from build123d import *

# Parameters (mm, degrees)
PAD_DEPTH       = 10
PAD003_DEPTH    = 12
POCKET_DEPTH    = 10
PAD004_DEPTH    = 12
POCKET004_DEPTH = 2
POCKET001_DEPTH = 10.001
SKETCH004_W     = 160
SKETCH004_H     = 60
PAD002_DEPTH    = 10
SKETCH005_W     = 156
SKETCH005_H     = 56
PAD005_DEPTH    = 12
SKETCH009_W     = 152
SKETCH009_H     = 52
POCKET006_DEPTH = 10
SKETCH006_W     = 18
SKETCH006_H     = 12
POCKET005_DEPTH = 10


with BuildPart() as part:
    # Sketch001 → Pad (new body)
    with BuildSketch(Plane.XY):
        with BuildLine():
            ThreePointArc((0, 57.236352), (-106.486482, 50.845622), (-101.68, -55.72412))
            Line((-101.68, -55.72412), (0, -150.0248))
            Line((0, -150.0248), (101.68, -55.72412))
            ThreePointArc((101.68, -55.72412), (106.486482, 50.845622), (0, 57.236352))
        make_face()
    extrude(amount=PAD_DEPTH)

    # Sketch002 → Pad003 (join)
    with BuildSketch(Plane.XY):
        with BuildLine():
            ThreePointArc((0, 54.552727), (-104.405447, 50.160217), (-100.32, -54.257696))
            Line((-100.32, -54.257696), (0, -147.297076))
            Line((0, -147.297076), (100.32, -54.257696))
            ThreePointArc((100.32, -54.257696), (104.405447, 50.160217), (0, 54.552727))
        make_face()
    extrude(amount=PAD003_DEPTH)

    # Sketch007 → Pocket (cut)
    with BuildSketch(Plane.XY.offset(12)):
        with BuildLine():
            ThreePointArc((0, 51.807335), (-102.301889, 49.482446), (-98.96, -52.791272))
            Line((-98.96, -52.791272), (0, -144.569352))
            Line((0, -144.569352), (98.96, -52.791272))
            ThreePointArc((98.96, -52.791272), (102.301889, 49.482446), (0, 51.807335))
        make_face()
    extrude(amount=-POCKET_DEPTH, mode=Mode.SUBTRACT)

    # Sketch008 → Pad004 (join)
    with BuildSketch(Plane.XY):
        with BuildLine():
            ThreePointArc((0, 33.166248), (-88.852758, 45.721583), (-90.8, -43.992727))
            Line((-90.8, -43.992727), (0, -128.203011))
            Line((0, -128.203011), (90.8, -43.992727))
            ThreePointArc((90.8, -43.992727), (88.852758, 45.721583), (0, 33.166248))
        make_face()
    extrude(amount=PAD004_DEPTH)

    # Sketch003 → Pocket004 (cut)
    with BuildSketch(Plane.XY.offset(12)):
        with BuildLine():
            ThreePointArc((0, 29.393877), (-86.345652, 45.199486), (-89.44, -42.526302))
            Line((-89.44, -42.526302), (0, -125.475287))
            Line((0, -125.475287), (89.44, -42.526302))
            ThreePointArc((89.44, -42.526302), (86.345652, 45.199486), (0, 29.393877))
        make_face()
    extrude(amount=-POCKET004_DEPTH, mode=Mode.SUBTRACT)

    # Sketch → Pocket001 (cut, through all)
    with BuildSketch(Plane.XY.offset(10)):
        with BuildLine():
            ThreePointArc((0, 25.21904), (-83.671135, 44.74656), (-88.08, -41.059878))
            Line((-88.08, -41.059878), (0, -122.747563))
            Line((0, -122.747563), (88.08, -41.059878))
            ThreePointArc((88.08, -41.059878), (83.671135, 44.74656), (0, 25.21904))
        make_face()
    extrude(amount=-POCKET001_DEPTH, mode=Mode.SUBTRACT)

    # Sketch004 → Pad002 (join)
    with BuildSketch(Plane.XY):
        with Locations((0, -170)):
            Rectangle(SKETCH004_W, SKETCH004_H)
    extrude(amount=PAD002_DEPTH)

    # Sketch005 → Pad005 (join)
    with BuildSketch(Plane.XY):
        with Locations((0, -170)):
            Rectangle(SKETCH005_W, SKETCH005_H)
    extrude(amount=PAD005_DEPTH)

    # Sketch009 → Pocket006 (cut)
    with BuildSketch(Plane.XY.offset(12)):
        with Locations((0, -170)):
            Rectangle(SKETCH009_W, SKETCH009_H)
    extrude(amount=-POCKET006_DEPTH, mode=Mode.SUBTRACT)

    # Sketch006 → Pocket005 (cut)
    with BuildSketch(Plane.XY.offset(12)):
        with Locations((0, -142.076699)):
            Rectangle(SKETCH006_W, SKETCH006_H)
    extrude(amount=-POCKET005_DEPTH, mode=Mode.SUBTRACT)


solid = part.part
For this review, take the finished solid that the model builds, in its own axes (mm). A direction names the side the tool comes from. Round coordinates to 2 decimals unless told otherwise and drop trailing zeros. Write each loop counter-clockwise with the first axis right and the second up, starting at its lowest first coordinate (ties: lowest second). Pieces come first, ordered by that corner, then holes. Notation, with made-up numbers: (76.25, 73.25) -> (90.25, 73.25) arc R20 ccw to (90.25, 92.25) -> close; hole circle Ø1 at (33, 88). An arc over 180 degrees is marked (long way). Use CSV: the item, a comma, the result in double quotes.
(1) Clearance check with flat-ended pins moving along their axes: P1, Ø5, axis at x = -47, z = 3, coming from the +Y side; P2, Ø5, axis at y = -128, z = 6, coming from the -X side; P3, Ø5, axis at y = -108, z = 10, coming from the -X side. State where each tip first meets the part, or that it passes through.
Computed values:
P1,"y = 76"
P2,"x = -26.44"
P3,"x = -48.01"
(2) Consider section C-C, the plane x = 15. Give the number of separate pieces and of enclosed holes in the cut face, plus the area to 3 significant figures.
Computed values:
separate pieces,"3"
enclosed holes,"0"
area,"478 mm²"
(3) Consider section B-B, the plane z = 4.25. Give the boundary of the cut face in (x, y).
Computed values:
outline,"(-101.68, -55.72) -> (-10.81, -140) -> (-80, -140) -> (-80, -200) -> (80, -200) -> (80, -140) -> (10.81, -140) -> (101.68, -55.72) arc R76 ccw to (0, 57.24) arc R76 ccw to start; (-90.8, -43.99) -> (0, -128.2) -> (90.8, -43.99) arc R60 ccw (long way) to (0, 33.17) arc R60 ccw (long way) to start; hole (-98.96, -52.79) -> (-9, -136.22) -> (-9, -144) -> (-76, -144) -> (-76, -196) -> (76, -196) -> (76, -144) -> (9, -144) -> (9, -136.22) -> (98.96, -52.79) arc R72 ccw (long way) to (0, 51.81) arc R72 ccw (long way) to start; hole (-88.08, -41.06) -> (0, -122.75) -> (88.08, -41.06) arc R56 ccw (long way) to (0, 25.22) arc R56 ccw (long way) to start"
(4) To check wall thickness, follow L1, parallel to X at y = 0, z = 5.75; L2, parallel to X at y = 0, z = 11.55; L3, parallel to Y at x = -59, z = 6.5. State the ranges of each line that lie inside material, in increasing order. Write a range as [from, to].
Computed values:
L1,"[-126, -122], [-110, -106], [106, 110], [122, 126]"
L2,"[-124, -122], [-110, -108], [108, 110], [122, 124]"
L3,"[-200, -196], [-144, -140], [-95.31, -89.85], [-73.48, -68.03], [55.27, 59.32], [71.44, 75.47]"
(5) Draft analysis for pull direction X (two halves, no side actions). For faces 1 (the face through (-45.346, -83.42, 11.014)), 2 (the face through (55.61, -98.45, 4.93)), 3 (the face through (-1, -200, 5)), state which applies: +X half, -X half, draft (parallel to the pull), parting line (faces both ways), or undercut.
Computed values:
face 1,"undercut"
face 2,"+X half"
face 3,"draft"
(6) Consider section A-A, the plane y = 0. Give the boundary of the cut face in (x, z), plus the area to 3 significant figures.
Computed values:
outline,"(-126, 0) -> (-106, 0) -> (-106, 10) -> (-108, 10) -> (-108, 12) -> (-110, 12) -> (-110, 2) -> (-122, 2) -> (-122, 12) -> (-124, 12) -> (-124, 10) -> (-126, 10) -> close; (106, 0) -> (126, 0) -> (126, 10) -> (124, 10) -> (124, 12) -> (122, 12) -> (122, 2) -> (110, 2) -> (110, 12) -> (108, 12) -> (108, 10) -> (106, 10) -> close"
area,"224 mm²"
(7) For faces 4 (the face through (84.756, 43.909, 5.07)), 5 (the face through (-54.61, -93.92, 7.07)), 6 (the face through (-56.881, -97.272, 4.93)), list the 3-axis set-ups (+Z, -Z, +X, -X, +Y, -Y) from which the entire face can be reached by the end or side of a thin tool; tool diameter is ignored.
Computed values:
face 4,"+Z, -Z"
face 5,"+Z"
face 6,"+Z, -Z, -X"
